The listing builds one solid part. Answer for the finished solid, in the listing's coordinates (mm). Coordinates: 2 decimals unless noted, no trailing zeros. Loops run counter-clockwise (first coordinate to the right, second up) from the corner with the lowest first, then second, coordinate; pieces in that order, holes last. Notation, with made-up numbers: (-27, -25) - (-12, -25) arc R16 ccw to (-12, 0) - close; hole circle Ø7 at (-6, 84). An arc over 180 degrees is marked (long way). Write each question's results on one line, items separated by ' | '. Start each with the question number.
(1) Find section B-B on z = -157.5. Determine the outline of the cut face in (x, y), then the cut area to 3 significant figures.
(2) Consider line 1 (X direction, y = 6.25, z = -161); line 2 (X direction, y = 3, z = -111); line 3 (Z direction, x = 241.5, y = 9). Determine where each line is inside the solid, lowest interval first. Write a range as from..to.
(3) Find section A-A on y = 8.5. State how many separate pieces and enclosed holes the cut face has, then the cut area to 3 significant figures.
(4) Find section C-C on x = 49. Determine the outline of the cut face in (y, z).
(5) Given pin 1 Ø3.5 at (x, z) = (276, -111) entering from -Y; pin 2 Ø7 at (x, z) = (280, -10) entering from +Y, each flat-ended and moving along its own axis, determine where each tip first touches the part or whether it passes through.
from build123d import *

# Parameters (mm, degrees)
ESQUISSE2_W             = 290
ESQUISSE2_H             = 290
ESQUISSE2_R             = 2
BOSS_EXTRU_1_DEPTH      = 10
ESQUISSE3_R             = 2
ENL_V_MAT_EXTRU_1_DEPTH = 10
CONG_1_R                = 10
ESQUISSE4_R             = 6
ENL_V_MAT_EXTRU_2_DEPTH = 5
ESQUISSE5_R             = 2
ENL_V_MAT_EXTRU_3_DEPTH = 10


with BuildPart() as part:
    # Esquisse2 → Boss.-Extru.1 (new body)
    with BuildSketch(Plane(origin=(0, 0, 0), x_dir=(1, 0, 0), z_dir=(0, 1, 0))):
        with Locations((145, 145)):
            Rectangle(ESQUISSE2_W, ESQUISSE2_H)
        with Locations((276, 111)):
            Circle(ESQUISSE2_R, mode=Mode.SUBTRACT)
        with Locations((225, 127)):
            Circle(ESQUISSE2_R, mode=Mode.SUBTRACT)
        with Locations((252, 221)):
            Circle(ESQUISSE2_R, mode=Mode.SUBTRACT)
        with Locations((14, 111)):
            Circle(ESQUISSE2_R, mode=Mode.SUBTRACT)
        with Locations((65, 127)):
            Circle(ESQUISSE2_R, mode=Mode.SUBTRACT)
        with Locations((38, 221)):
            Circle(ESQUISSE2_R, mode=Mode.SUBTRACT)
        Polygon((233, 185), (233, 145), (233, 105), (260, 105), (260, 120), (280, 120), (280, 185), align=None, mode=Mode.SUBTRACT)
        Polygon((30, 105), (30, 120), (10, 120), (10, 185), (57, 185), (57, 145), (57, 105), align=None, mode=Mode.SUBTRACT)
    extrude(amount=BOSS_EXTRU_1_DEPTH)

    # Esquisse3 → Enlèv. mat.-Extru.1 (cut)
    with BuildSketch(Plane(origin=(0, 10, 0), x_dir=(1, 0, 0), z_dir=(0, 1, 0))):
        with Locations((10, 280)):
            Circle(ESQUISSE3_R)
        with Locations((280, 280)):
            Circle(ESQUISSE3_R)
        with Locations((280, 10)):
            Circle(ESQUISSE3_R)
        with Locations((10, 10)):
            Circle(ESQUISSE3_R)
    extrude(amount=-ENL_V_MAT_EXTRU_1_DEPTH, mode=Mode.SUBTRACT)

    # Congé1
    cong_1_edges = [part.edges().sort_by_distance(p)[0] for p in [
        (0, 5, -290),
        (290, 5, -290),
        (290, 5, 0),
        (0, 5, 0),
    ]]
    fillet(cong_1_edges, radius=CONG_1_R)

    # Esquisse4 → Enlèv. mat.-Extru.2 (cut)
    with BuildSketch(Plane(origin=(0, 10, 0), x_dir=(1, 0, 0), z_dir=(0, 1, 0))):
        with Locations((10, 280)):
            Circle(ESQUISSE4_R)
        with Locations((280, 280)):
            Circle(ESQUISSE4_R)
        with Locations((280, 10)):
            Circle(ESQUISSE4_R)
        with Locations((10, 10)):
            Circle(ESQUISSE4_R)
    extrude(amount=-ENL_V_MAT_EXTRU_2_DEPTH, mode=Mode.SUBTRACT)

    # Esquisse5 → Enlèv. mat.-Extru.3 (cut)
    with BuildSketch(Plane.XZ):
        with Locations((102, -14)):
            Circle(ESQUISSE5_R)
        with Locations((188, -14)):
            Circle(ESQUISSE5_R)
        with Locations((188, -100)):
            Circle(ESQUISSE5_R)
        with Locations((102, -100)):
            Circle(ESQUISSE5_R)
    extrude(amount=-ENL_V_MAT_EXTRU_3_DEPTH, mode=Mode.SUBTRACT)


solid = part.part
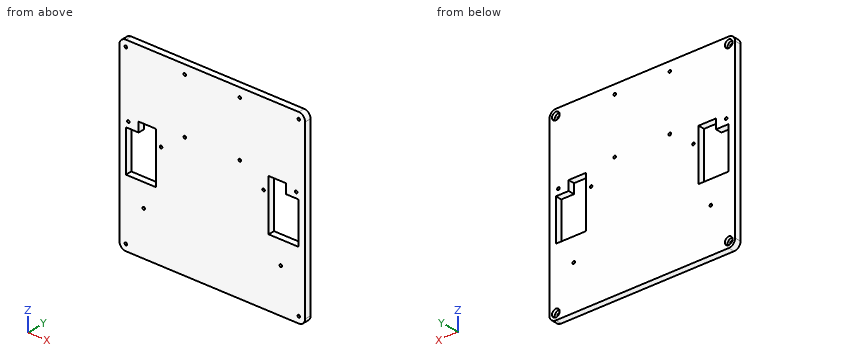
Values:
1) outline: (0, 0) - (10, 0) - (10, 10) - (0, 10) - close; (57, 0) - (233, 0) - (233, 10) - (57, 10) - close; (280, 0) - (290, 0) - (290, 10) - (280, 10) - close | area: 1,960 mm²
2) line 1: x = 0..10, 57..233, 280..290 | line 2: x = 0..12, 16..30, 57..233, 260..274, 278..290 | line 3: z = -290..-185, -105..0
3) separate pieces: 1 | enclosed holes: 16 | area: 76,500 mm²
4) outline: (0, -290) - (10, -290) - (10, -185) - (0, -185) - close; (0, -105) - (10, -105) - (10, 0) - (0, 0) - close
5) pin 1: passes through | pin 2: stops at y = 5
